from build123d import *

# Parameters (mm, degrees)
CROQUIS1_R                 = 17.5
SALIENTE_EXTRUIR1_DEPTH    = 12
CROQUIS2_W                 = 15
CROQUIS2_H                 = 8
SALIENTE_EXTRUIR2_DEPTH    = 38
CROQUIS3_W                 = 15
CROQUIS3_H                 = 8
SALIENTE_EXTRUIR3_DEPTH    = 15
REDONDEO1_RADIUS           = 7.5
REDONDEO1_LENGTH           = 8
CROQUIS4_R                 = 6.6
CORTAR_EXTRUIR1_DEPTH      = 5.2
CORTAR_EXTRUIR2_START      = -5.2
CROQUIS5_R                 = 6.6
CORTAR_EXTRUIR2_DEPTH      = 5.2
CROQUIS7_R                 = 5
SALIENTE_EXTRUIR4_DEPTH    = 1.5
CORTAR_EXTRUIR3_DEPTH      = 58.089841478
CORTAR_EXTRUIR3_DEPTH_BACK = 58.089841478
CROQUIS6_R                 = 1.6


with BuildPart() as part:
    # Croquis1 → Saliente-Extruir1 (new body)
    with BuildSketch(Plane.XY):
        Circle(CROQUIS1_R)
    extrude(amount=SALIENTE_EXTRUIR1_DEPTH)

    # Croquis2 → Saliente-Extruir2 (add)
    with BuildSketch(Plane(origin=(0, 0, 0), x_dir=(1, 0, 0), z_dir=(0, 1, 0))):
        with Locations((0, -4)):
            Rectangle(CROQUIS2_W, CROQUIS2_H)
    extrude(amount=SALIENTE_EXTRUIR2_DEPTH)

    # Croquis3 → Saliente-Extruir3 (add)
    with BuildSketch(Plane(origin=(0, 38, 0), x_dir=(1, 0, 0), z_dir=(0, 1, 0))):
        with Locations((0, -4)):
            Rectangle(CROQUIS3_W, CROQUIS3_H)
    extrude(amount=SALIENTE_EXTRUIR3_DEPTH)

    # Redondeo1: full round fillet: the end face becomes a half cylinder, R = half its width
    redondeo1_face = Plane((0, 53, 4), x_dir=(0, 0, 1), z_dir=(0, 1, 0))  # on the end face: x along it, z out of the body
    redondeo1_slab = redondeo1_face.offset(-REDONDEO1_RADIUS / 2) * Box(REDONDEO1_LENGTH, 2 * REDONDEO1_RADIUS, REDONDEO1_RADIUS, mode=Mode.PRIVATE)  # the body's end, R deep
    redondeo1_round = Plane((0, 45.5, 4), x_dir=(0, 1, 0), z_dir=(0, 0, 1)) * Cylinder(REDONDEO1_RADIUS, REDONDEO1_LENGTH, mode=Mode.PRIVATE)  # its axis R under the face
    add(redondeo1_slab - redondeo1_round, mode=Mode.SUBTRACT)

    # Croquis4 → Cortar-Extruir1 (cut)
    with BuildSketch(Plane.XY.offset(12)):
        Circle(CROQUIS4_R)
    extrude(amount=-CORTAR_EXTRUIR1_DEPTH, mode=Mode.SUBTRACT)

    # Croquis5 → Cortar-Extruir2 (cut)
    with BuildSketch(Plane(origin=(0, 0, 0), x_dir=(-1, 0, 0), z_dir=(0, 0, -1)).offset(CORTAR_EXTRUIR2_START)):
        with Locations(Location((0, 0, 0), (0, 0, 180))):
            Circle(CROQUIS5_R)
    extrude(amount=CORTAR_EXTRUIR2_DEPTH, mode=Mode.SUBTRACT)

    # Croquis7 → Saliente-Extruir4 (add)
    with BuildSketch(Plane(origin=(0, 0, 0), x_dir=(-1, 0, 0), z_dir=(0, 0, -1))):
        with Locations(Location((0, 45.5, 0), (0, 0, 180))):
            Circle(CROQUIS7_R)
    extrude(amount=SALIENTE_EXTRUIR4_DEPTH)

    # Croquis6 → Cortar-Extruir3 (cut, two sides: drawn at the far end of the back side and taken through both)
    with BuildSketch(Plane(origin=(0, 0, 0), x_dir=(-1, 0, 0), z_dir=(0, 0, -1)).offset(-CORTAR_EXTRUIR3_DEPTH_BACK)):
        with Locations((0, 45.5)):
            Circle(CROQUIS6_R)
    extrude(amount=CORTAR_EXTRUIR3_DEPTH + CORTAR_EXTRUIR3_DEPTH_BACK, mode=Mode.SUBTRACT)


solid = part.part
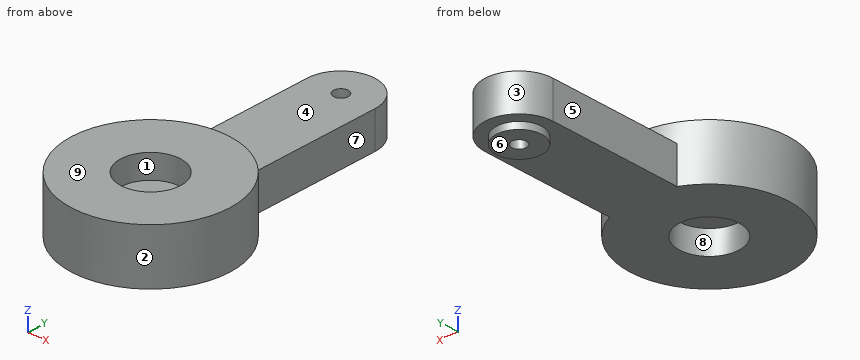
The listing builds one solid part. Answer for the finished solid, in the listing's coordinates (mm). Face numbers are marked on the shaded views. A direction names the side the tool comes from. Give positions to 0.01 mm unless a question says otherwise; leave off trailing zeros. Order: outer loops, then holes, each group sorted by start corner. A loop starts at its lowest first (then second) coordinate and runs counter-clockwise, first axis right, second up. Notation, with made-up numbers: (56, -8) - (73, -8) arc R20 cw to (73, 29) - close; hole circle Ø5 at (1.25, 45.5). An arc over 180 degrees is marked (long way). One line per item, written item: value. Start each with the question number.
1) A cutting plane is placed at D-D on z = 8.75. Give the vertices of the cut face in (x, y), then the cut area to 3 significant figures.
2) A cutting plane is placed at C-C on z = 2. Give the vertices of the cut face in (x, y), then the cut area to 3 significant figures.
3) The mould has two halves that part along Y. Classify the marked faces 1, 2, 3 and 4: released by +Y, released by -Y, zero draft, split by the parting line, or undercut.
4) A cutting plane is placed at A-A on x = 0. Give the vertices of the cut face in (y, z), then the cut area to 3 significant figures.
5) Find the intervals of material crossed by L1, parallel to Y at x = 0, z = 2.15; L2, parallel to Y at x = 0, z = 5.75; L3, parallel to Y at x = 0, z = 8.15, in increasing order.
6) A cutting plane is placed at B-B on y = 0. Give the vertices of the cut face in (x, z), then the cut area to 3 significant figures.
7) Given pin 1 Ø4 at (y, z) = (36, 2.5) entering from +X; pin 2 Ø12 at (x, y) = (0, 42) entering from +Z; pin 3 Ø4 at (x, z) = (-10, 7) entering from -Y, each flat-ended and moving along its own axis, determine where each tip first touches the part or whether it passes through.
8) A tool of negligible diameter and unlimited length cuts with its end or side. For the marked faces 5, 6, 7, 8 and 9, from which of +Z, -Z, +X, -X, +Y, -Y can it reach the whole face along a straight path? Write none if from no direction.
Answer sheet:
1. outline: circle Ø35 at (0, 0); hole circle Ø13.2 at (0, 0)
1. area: 825 mm2
2. outline: (-7.5, 15.81) arc R17.5 ccw (long way) to (7.5, 15.81) - (7.5, 45.5) arc R7.5 ccw to (-7.5, 45.5) - close; hole circle Ø13.2 at (0, 0); hole circle Ø3.2 at (0, 45.5)
2. area: 1,330 mm2
3. face 1: undercut
3. face 2: split by the parting line
3. face 3: released by +Y
3. face 4: zero draft
4. outline: (-17.5, 0) - (-6.6, 0) - (-6.6, 5.2) - (6.6, 5.2) - (6.6, 0) - (40.5, 0) - (40.5, -1.5) - (43.9, -1.5) - (43.9, 8) - (17.5, 8) - (17.5, 12) - (6.6, 12) - (6.6, 6.8) - (-6.6, 6.8) - (-6.6, 12) - (-17.5, 12) - close; (47.1, -1.5) - (50.5, -1.5) - (50.5, 0) - (53, 0) - (53, 8) - (47.1, 8) - close
4. area: 551 mm2
5. L1: y = -17.5 to -6.6, 6.6 to 43.9, 47.1 to 53
5. L2: y = -17.5 to 43.9, 47.1 to 53
5. L3: y = -17.5 to -6.6, 6.6 to 17.5
6. outline: (-17.5, 0) - (-6.6, 0) - (-6.6, 5.2) - (6.6, 5.2) - (6.6, 0) - (17.5, 0) - (17.5, 12) - (6.6, 12) - (6.6, 6.8) - (-6.6, 6.8) - (-6.6, 12) - (-17.5, 12) - close
6. area: 283 mm2
7. pin 1: stops at x = 7.5
7. pin 2: stops at z = 8
7. pin 3: stops at y = -15.56
8. face 5: +Z, -Z, -X, +Y
8. face 6: -Z, +X, -X, +Y, -Y
8. face 7: +Z, -Z, +X, +Y
8. face 8: -Z
8. face 9: +Z, +X, -X, +Y, -Y
